Geometry check sheet. Reference: the model listing, model coordinates, mm. Face numbers are marked on the shaded views. A direction names the side the tool comes from. Round coordinates to 2 decimals unless told otherwise and drop trailing zeros. Write each loop counter-clockwise with the first axis right and the second up, starting at its lowest first coordinate (ties: lowest second). Pieces come first, ordered by that corner, then holes. Notation, with made-up numbers: (72.25, 87.5) -> (92.25, 87.5) arc R14 ccw to (92.25, 113.5) -> close; hole circle Ø1 at (45, 74.25). An arc over 180 degrees is marked (long way). Use a Markdown table: item, result.
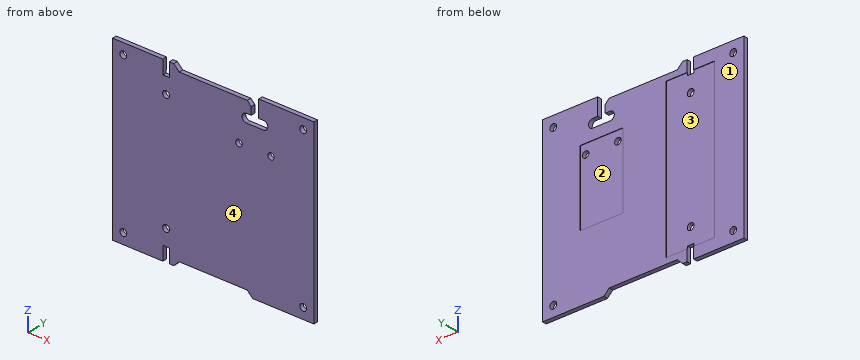
```python
from build123d import *

# Parameters (mm, degrees)
SKETCH1_W           = 94
SKETCH1_H           = 83
SKETCH1_R           = 1.5875
BOSS_EXTRUDE1_DEPTH = 2
SKETCH2_R           = 1.6
SKETCH2_R_2         = 1.5
SKETCH2_W           = 3
SKETCH2_H           = 6.5
CUT_EXTRUDE1_DEPTH  = 3
SKETCH3_W           = 22.5
SKETCH3_H           = 72.5
SKETCH3_W_2         = 20
SKETCH3_H_2         = 35
CUT_EXTRUDE2_DEPTH  = 0.2
CUT_EXTRUDE3_DEPTH  = 3


with BuildPart() as part:
    # Sketch1 → Boss-Extrude1 (new body)
    with BuildSketch(Plane(origin=(0, 0, 0), x_dir=(1, 0, 0), z_dir=(0, 1, 0))):
        Rectangle(SKETCH1_W, SKETCH1_H)
        with Locations((-42, 36.5)):
            Circle(SKETCH1_R, mode=Mode.SUBTRACT)
        with Locations((42, 36.5)):
            Circle(SKETCH1_R, mode=Mode.SUBTRACT)
        with Locations((42, -36.5)):
            Circle(SKETCH1_R, mode=Mode.SUBTRACT)
        with Locations((-42, -36.5)):
            Circle(SKETCH1_R, mode=Mode.SUBTRACT)
    extrude(amount=BOSS_EXTRUDE1_DEPTH)

    # Sketch2 → Cut-Extrude1 (cut, through all)
    with BuildSketch(Plane(origin=(0, 2, 0), x_dir=(1, 0, 0), z_dir=(0, 1, 0))):
        with Locations((-22, -27.5)):
            Circle(SKETCH2_R)
        with Locations((-22, 27.5)):
            Circle(SKETCH2_R)
        with Locations((12, -20)):
            Circle(SKETCH2_R_2)
        with Locations((27, -20)):
            Circle(SKETCH2_R_2)
        with Locations((-22, 38.25)):
            Rectangle(SKETCH2_W, SKETCH2_H)
        with Locations((-22, -38.25)):
            Rectangle(SKETCH2_W, SKETCH2_H)
        with BuildLine():
            Line((15.5, -29.5), (23.5, -29.5))
            ThreePointArc((23.5, -29.5), (25.5, -31.5), (23.5, -33.5))
            Line((23.5, -33.5), (21.25, -33.5))
            Line((21.25, -33.5), (21.25, -41.5))
            Line((21.25, -41.5), (17.75, -41.5))
            Line((17.75, -41.5), (17.75, -33.5))
            Line((17.75, -33.5), (15.5, -33.5))
            ThreePointArc((15.5, -33.5), (13.5, -31.5), (15.5, -29.5))
        make_face()
    extrude(amount=-CUT_EXTRUDE1_DEPTH, mode=Mode.SUBTRACT)

    # Sketch3 → Cut-Extrude2 (cut)
    with BuildSketch(Plane(origin=(0, 2, 0), x_dir=(1, 0, 0), z_dir=(0, 1, 0))):
        with Locations((-22, 0)):
            Rectangle(SKETCH3_W, SKETCH3_H)
        with Locations((19.5, -7)):
            Rectangle(SKETCH3_W_2, SKETCH3_H_2)
    extrude(amount=-CUT_EXTRUDE2_DEPTH, mode=Mode.SUBTRACT)

    # Sketch4 → Cut-Extrude3 (cut, through all)
    with BuildSketch(Plane(origin=(0, 2, 0), x_dir=(1, 0, 0), z_dir=(0, 1, 0))):
        Polygon((18.415, 41.5), (-18.415, 41.5), (-15.875, 38.96), (15.875, 38.96), align=None)
        Polygon((-15.875, -38.96), (-18.415, -41.5), (17.75, -41.5), (17.75, -37.085), (15.875, -38.96), align=None)
    extrude(amount=-CUT_EXTRUDE3_DEPTH, mode=Mode.SUBTRACT)


solid = part.part
```
(1) Thickness scan on line 1 (Z direction, x = -22, y = 0.6); line 2 (Z direction, x = -42, y = 0.55); line 3 (X direction, y = 1.45, z = -36.5). Record the ranges inside material, lowest first.
A:
| item | result |
|---|---|
| line 1 | z = -35 to -29.1, -25.9 to 25.9, 29.1 to 35 |
| line 2 | z = -41.5 to -38.09, -34.91 to 34.91, 38.09 to 41.5 |
| line 3 | x = -47 to -43.59, -40.41 to -23.5, -20.5 to 40.41, 43.59 to 47 |
(2) Section check A-A on x = 42. Record the cut outline in (y, z), plus the area to 3 significant figures.
A:
| item | result |
|---|---|
| outline | (0, -41.5) -> (2, -41.5) -> (2, -38.09) -> (0, -38.09) -> close; (0, -34.91) -> (2, -34.91) -> (2, 34.91) -> (0, 34.91) -> close; (0, 38.09) -> (2, 38.09) -> (2, 41.5) -> (0, 41.5) -> close |
| area | 153 mm2 |
(3) Section check B-B on z = 27.5. Record the cut outline in (x, y).
A:
| item | result |
|---|---|
| outline | (-47, 0) -> (-23.6, 0) -> (-23.6, 1.8) -> (-33.25, 1.8) -> (-33.25, 2) -> (-47, 2) -> close; (-20.4, 0) -> (47, 0) -> (47, 2) -> (-10.75, 2) -> (-10.75, 1.8) -> (-20.4, 1.8) -> close |
(4) Release check for a two-part mould opening along Z. For the marked faces 3 and 4 record: +Z half, -Z half, draft (parallel to the pull), parting line (faces both ways), or undercut.
A:
| item | result |
|---|---|
| face 3 | undercut |
| face 4 | draft |
(5) Gauge pin test, flat ends, axial feed: pin 1 Ø4 at (x, z) = (-22, -27.5) entering from -Y; pin 2 Ø5 at (x, z) = (-22, 27.5) entering from +Y; pin 3 Ø3 at (x, z) = (42, 36.5) entering from -Y; pin 4 Ø0.6 at (x, y) = (19, 1) entering from +Z. Record the tip position at first contact, or that the pin passes through.
A:
| item | result |
|---|---|
| pin 1 | stops at y = 0 |
| pin 2 | stops at y = 1.8 |
| pin 3 | passes through |
| pin 4 | stops at z = 29.5 |
(6) Section check D-D on z = -6.5. Record the cut outline in (x, y), plus the area to 4 significant figures.
A:
| item | result |
|---|---|
| outline | (-47, 0) -> (47, 0) -> (47, 2) -> (29.5, 2) -> (29.5, 1.8) -> (9.5, 1.8) -> (9.5, 2) -> (-10.75, 2) -> (-10.75, 1.8) -> (-33.25, 1.8) -> (-33.25, 2) -> (-47, 2) -> close |
| area | 179.5 mm2 |
(7) Section check C-C on x = 27. Record the cut outline in (y, z).
A:
| item | result |
|---|---|
| outline | (0, -41.5) -> (2, -41.5) -> (2, -10.5) -> (1.8, -10.5) -> (1.8, 18.5) -> (0, 18.5) -> close; (0, 21.5) -> (1.8, 21.5) -> (1.8, 24.5) -> (2, 24.5) -> (2, 41.5) -> (0, 41.5) -> close |
(8) Access from +Z, -Z, +X, -X, +Y, -Y to the whole of each face (thin tool, end or side, straight path). Record for the marked faces 1 and 2.
A:
| item | result |
|---|---|
| face 1 | +Z, -Z, +X, -X, +Y |
| face 2 | +Y |
